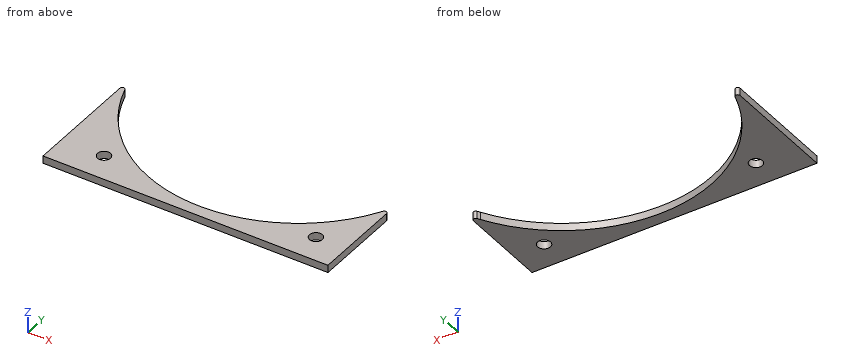
Autodesk Inventor part; units mm, degrees
ref_plane "YZ Plane" through (0, 0, 0) normal (1, 0, 0) x (0, 1, 0)
ref_plane "XZ Plane" through (0, 0, 0) normal (0, 1, 0) x (-1, 0, 0)
ref_plane "XY Plane" through (0, 0, 0) normal (0, 0, 1) x (1, 0, 0)
sketch "Sketch1" plane through (0, 0, 0) normal (0, 0, 1) x (1, 0, 0)
  arc A0 (-17, -31.2731) -> (-18.866, -30.7731) centre (-18, -31.2731) ccw
  line L0 (-17, -31.2731) -> (-17, -69)
  line L1 (-17, -69) -> (-138, -69)
  line L2 (-138, -69) -> (-138, -19.5192)
  arc A1 (-136.0462, -19.2189) -> (-138, -19.5192) centre (-137, -19.5192) ccw
  arc A2 (-136.0462, -19.2189) -> (-19.5744, -32) centre (-75, 0) ccw
  line L3 (-19.5744, -32) -> (-18.866, -30.7731)
  circle A3 centre (-30, -57) radius 2.75
  circle A4 centre (-120, -57) radius 2.75
  line L4 (-138, -69) -> (-17, -69)
  arc A5 (-17, -31.2731) -> (-18.866, -30.7731) centre (-18, -31.2731) ccw
  line L5 (-17, -31.2731) -> (-17, -69)
  line L6 (-17, -69) -> (-138, -69)
  line L7 (-138, -69) -> (-138, -19.5192)
  arc A6 (-136.0462, -19.2189) -> (-138, -19.5192) centre (-137, -19.5192) ccw
  arc A7 (-136.0462, -19.2189) -> (-19.5744, -32) centre (-75, 0) ccw
  line L8 (-19.5744, -32) -> (-18.866, -30.7731)
  circle A8 centre (-30, -57) radius 2.75
  circle A9 centre (-120, -57) radius 2.75
  point P0 (0, 0)
extrude "Extrusion1" add sketch "Sketch1" along normal blind 3.175
properties part number "1-8inch_Sieve_Piece1"
Input: part model. Units: mm. Frame: model coordinates. Give positions to 0.01 mm unless a question says otherwise; leave off trailing zeros. Order: outer loops, then holes, each group sorted by start corner. A loop starts at its lowest first (then second) coordinate and runs counter-clockwise, first axis right, second up. Notation, with made-up numbers: (23.5, 42) - (72.5, 42) arc R35 ccw to (72.5, 77) - close; hole circle Ø8 at (36.5, 74). An arc over 180 degrees is marked (long way). Use a Markdown table: item, result.
(1) Section query C-C (x = -28.5). Output: boundary loops of the cut face in (y, z) (3 decimals), then the cut area to 3 significant figures.
Computed values:
| item | result |
|---|---|
| outline | (-69, 0) - (-59.305, 0) - (-59.305, 3.175) - (-69, 3.175) - close; (-54.695, 0) - (-43.974, 0) - (-43.974, 3.175) - (-54.695, 3.175) - close |
| area | 64.8 mm2 |
(2) Section query B-B (z = 2.35). Output: boundary loops of the cut face in (x, y).
Computed values:
| item | result |
|---|---|
| outline | (-138, -69) - (-17, -69) - (-17, -31.27) arc R1 ccw to (-18.87, -30.77) - (-19.57, -32) arc R64 cw to (-136.05, -19.22) arc R1 ccw to (-138, -19.52) - close; hole circle Ø5.5 at (-120, -57); hole circle Ø5.5 at (-30, -57) |
(3) Line query: line 1 (X direction, y = -34, z = 2.45); line 2 (Y direction, x = -30, z = 0.95); line 3 (X direction, y = -40, z = 0.65). Output: solid intervals per line, ascending. Write a range as from..to.
Computed values:
| item | result |
|---|---|
| line 1 | x = -138..-129.22, -20.78..-17 |
| line 2 | y = -69..-59.75, -54.25..-45.51 |
| line 3 | x = -138..-124.96, -25.04..-17 |
(4) Pin query (flat end, axial travel): pin 1 (1 mm diameter, centred on x = -107.5, z = 3, fed in from +Y). Return the tip coordinate at first contact, or that it passes through.
Computed values:
| item | result |
|---|---|
| pin 1 | stops at y = -54.84 |
(5) Section query D-D (x = -57.5). Output: boundary loops of the cut face in (y, z) (3 decimals), then the cut area to 3 significant figures.
Computed values:
| item | result |
|---|---|
| outline | (-69, 0) - (-61.561, 0) - (-61.561, 3.175) - (-69, 3.175) - close |
| area | 23.6 mm2 |
(6) Section query A-A (y = -40). Output: boundary loops of the cut face in (x, z) (3 decimals).
Computed values:
| item | result |
|---|---|
| outline | (-138, 0) - (-124.96, 0) - (-124.96, 3.175) - (-138, 3.175) - close; (-25.04, 0) - (-17, 0) - (-17, 3.175) - (-25.04, 3.175) - close |
